from build123d import *

# Parameters (mm, degrees)
F0_R     = 25.4
F0_R_2   = 3.125
F1_DEPTH = 5
F2_R     = 6.031593
F3_DEPTH = 8
F4_R     = 3
F5_DEPTH = 8.001
F8_R     = 1.008959
F9_DEPTH = 8.001


with BuildPart() as f1:
    # F0 (on Top) → F1 (new body)
    with BuildSketch(Plane.XY):
        Circle(F0_R)
        with BuildLine():
            ThreePointArc((-10.88453, -17.158945), (-11.801786, -15.683608), (-11.218679, -14.04716))
            Line((-11.218679, -14.04716), (-6.139343, -9.030124))
            ThreePointArc((-6.139343, -9.030124), (-5.086026, -8.484282), (-3.908805, -8.631157))
            ThreePointArc((-3.908805, -8.631157), (-3.625926, -8.753759), (-3.339207, -8.867092))
            ThreePointArc((-3.339207, -8.867092), (-2.40293, -9.595657), (-2.044091, -10.726433))
            Line((-2.044091, -10.726433), (-2.000038, -17.865646))
            ThreePointArc((-2.000038, -17.865646), (-2.744862, -19.435109), (-4.436681, -19.829732))
            ThreePointArc((-4.436681, -19.829732), (-7.776127, -18.773232), (-10.88453, -17.158945))
        make_face(mode=Mode.SUBTRACT)
        with BuildLine():
            ThreePointArc((-19.829732, -4.436681), (-19.435109, -2.744862), (-17.865646, -2.000038))
            Line((-17.865646, -2.000038), (-10.726433, -2.044091))
            ThreePointArc((-10.726433, -2.044091), (-9.595657, -2.40293), (-8.867092, -3.339207))
            ThreePointArc((-8.867092, -3.339207), (-8.753759, -3.625926), (-8.631157, -3.908805))
            ThreePointArc((-8.631157, -3.908805), (-8.484282, -5.086026), (-9.030124, -6.139343))
            Line((-9.030124, -6.139343), (-14.04716, -11.218679))
            ThreePointArc((-14.04716, -11.218679), (-15.683608, -11.801786), (-17.158945, -10.88453))
            ThreePointArc((-17.158945, -10.88453), (-18.773232, -7.776127), (-19.829732, -4.436681))
        make_face(mode=Mode.SUBTRACT)
        Circle(F0_R_2, mode=Mode.SUBTRACT)
        with BuildLine():
            ThreePointArc((4.436681, -19.829732), (2.744862, -19.435109), (2.000038, -17.865646))
            Line((2.000038, -17.865646), (2.044091, -10.726433))
            ThreePointArc((2.044091, -10.726433), (2.40293, -9.595657), (3.339207, -8.867092))
            ThreePointArc((3.339207, -8.867092), (3.625926, -8.753759), (3.908805, -8.631157))
            ThreePointArc((3.908805, -8.631157), (5.086026, -8.484282), (6.139343, -9.030124))
            Line((6.139343, -9.030124), (11.218679, -14.04716))
            ThreePointArc((11.218679, -14.04716), (11.801786, -15.683608), (10.88453, -17.158945))
            ThreePointArc((10.88453, -17.158945), (7.776127, -18.773232), (4.436681, -19.829732))
        make_face(mode=Mode.SUBTRACT)
        with BuildLine():
            ThreePointArc((17.158945, -10.88453), (15.683608, -11.801786), (14.04716, -11.218679))
            Line((14.04716, -11.218679), (9.030124, -6.139343))
            ThreePointArc((9.030124, -6.139343), (8.484282, -5.086026), (8.631157, -3.908805))
            ThreePointArc((8.631157, -3.908805), (8.753759, -3.625926), (8.867092, -3.339207))
            ThreePointArc((8.867092, -3.339207), (9.595657, -2.40293), (10.726433, -2.044091))
            Line((10.726433, -2.044091), (17.865646, -2.000038))
            ThreePointArc((17.865646, -2.000038), (19.435109, -2.744862), (19.829732, -4.436681))
            ThreePointArc((19.829732, -4.436681), (18.773232, -7.776127), (17.158945, -10.88453))
        make_face(mode=Mode.SUBTRACT)
        with BuildLine():
            ThreePointArc((-17.158945, 10.88453), (-15.683608, 11.801786), (-14.04716, 11.218679))
            Line((-14.04716, 11.218679), (-9.030124, 6.139343))
            ThreePointArc((-9.030124, 6.139343), (-8.484282, 5.086026), (-8.631157, 3.908805))
            ThreePointArc((-8.631157, 3.908805), (-8.753759, 3.625926), (-8.867092, 3.339207))
            ThreePointArc((-8.867092, 3.339207), (-9.595657, 2.40293), (-10.726433, 2.044091))
            Line((-10.726433, 2.044091), (-17.865646, 2.000038))
            ThreePointArc((-17.865646, 2.000038), (-19.435109, 2.744862), (-19.829732, 4.436681))
            ThreePointArc((-19.829732, 4.436681), (-18.773232, 7.776127), (-17.158945, 10.88453))
        make_face(mode=Mode.SUBTRACT)
        with BuildLine():
            ThreePointArc((-10.88453, 17.158945), (-7.776127, 18.773232), (-4.436681, 19.829732))
            ThreePointArc((-4.436681, 19.829732), (-2.744862, 19.435109), (-2.000038, 17.865646))
            Line((-2.000038, 17.865646), (-2.044091, 10.726433))
            ThreePointArc((-2.044091, 10.726433), (-2.40293, 9.595657), (-3.339207, 8.867092))
            ThreePointArc((-3.339207, 8.867092), (-3.625926, 8.753759), (-3.908805, 8.631157))
            ThreePointArc((-3.908805, 8.631157), (-5.086026, 8.484282), (-6.139343, 9.030124))
            Line((-6.139343, 9.030124), (-11.218679, 14.04716))
            ThreePointArc((-11.218679, 14.04716), (-11.801786, 15.683608), (-10.88453, 17.158945))
        make_face(mode=Mode.SUBTRACT)
        with BuildLine():
            ThreePointArc((19.829732, 4.436681), (19.435109, 2.744862), (17.865646, 2.000038))
            Line((17.865646, 2.000038), (10.726433, 2.044091))
            ThreePointArc((10.726433, 2.044091), (9.595657, 2.40293), (8.867092, 3.339207))
            ThreePointArc((8.867092, 3.339207), (8.753759, 3.625926), (8.631157, 3.908805))
            ThreePointArc((8.631157, 3.908805), (8.484282, 5.086026), (9.030124, 6.139343))
            Line((9.030124, 6.139343), (14.04716, 11.218679))
            ThreePointArc((14.04716, 11.218679), (15.683608, 11.801786), (17.158945, 10.88453))
            ThreePointArc((17.158945, 10.88453), (18.773232, 7.776127), (19.829732, 4.436681))
        make_face(mode=Mode.SUBTRACT)
        with BuildLine():
            Line((2.044091, 10.726433), (2.000038, 17.865646))
            ThreePointArc((2.000038, 17.865646), (2.744862, 19.435109), (4.436681, 19.829732))
            ThreePointArc((4.436681, 19.829732), (7.776127, 18.773232), (10.88453, 17.158945))
            ThreePointArc((10.88453, 17.158945), (11.801786, 15.683608), (11.218679, 14.04716))
            Line((11.218679, 14.04716), (6.139343, 9.030124))
            ThreePointArc((6.139343, 9.030124), (5.086026, 8.484282), (3.908805, 8.631157))
            ThreePointArc((3.908805, 8.631157), (3.625926, 8.753759), (3.339207, 8.867092))
            ThreePointArc((3.339207, 8.867092), (2.40293, 9.595657), (2.044091, 10.726433))
        make_face(mode=Mode.SUBTRACT)
    extrude(amount=F1_DEPTH)

    # F2 (on Top) → F3 (join)
    with BuildSketch(Plane.XY):
        Circle(F2_R)
    extrude(amount=F3_DEPTH)

    # F4 (on face) → F5 (cut, through all)
    with BuildSketch(Plane.XY.offset(8)):
        Circle(F4_R)
    extrude(amount=-F5_DEPTH, mode=Mode.SUBTRACT)

    # F6 (on Right) → F7 (revolve, cut)
    with BuildSketch(Plane.YZ):
        Polygon((25.457971, 0.902619), (25.4, 2.402619), (23.4, 2.402619), align=None)
        Polygon((23.4, 2.402619), (25.4, 2.402619), (25.457971, 3.902619), align=None)
    revolve(axis=Axis((0, 0, 8.098846), (0, 0, -1)), mode=Mode.SUBTRACT)

    # F8 (on Top) → F9 (cut, through all)
    with BuildSketch(Plane.XY):
        with Locations((0, 4.377856)):
            Circle(F8_R)
        with Locations((-3.095612, 3.095612)):
            Circle(F8_R)
        with Locations((-4.377856, 0)):
            Circle(F8_R)
        with Locations((-3.095612, -3.095612)):
            Circle(F8_R)
        with Locations((0, -4.377856)):
            Circle(F8_R)
        with Locations((3.095612, -3.095612)):
            Circle(F8_R)
        with Locations((4.377856, 0)):
            Circle(F8_R)
        with Locations((3.095612, 3.095612)):
            Circle(F8_R)
    extrude(amount=F9_DEPTH, mode=Mode.SUBTRACT)


solid = f1.part
Verification items for the finished model (mm, model axes). Give positions to 0.01 mm unless a question says otherwise; leave off trailing zeros. Write each loop counter-clockwise with the first axis right and the second up, starting at its lowest first coordinate (ties: lowest second). Pieces come first, ordered by that corner, then holes. Notation, with made-up numbers: (47.25, 50) - (105.25, 50) arc R27 ccw to (105.25, 89) - close; hole circle Ø8 at (8.5, 79). An arc over 180 degrees is marked (long way). Answer as CSV lines item,"result". Start each with the question number.
1. Thickness scan on line 1 (Y direction, x = 0, z = 5.75); line 2 (Y direction, x = 7, z = 2.25); line 3 (Y direction, x = 14, z = 3.25). Record the ranges inside material, lowest first.
2. Sectioned sample at C-C (z = 6.5). Count the separate pieces of the cut face and the enclosed holes in it, then the cut area to 3 significant figures.
3. Draft check along Y on faces 1 (the face through (-11.57, 8.71, 2.46)), 2 (the face through (5, -5, 5)), 3 (the face through (-5.506, -24.796, 4.422)). Enter one of: pulls with the +Y half, pulls with the -Y half, needs draft (parallel to the pull), parting line crosses it, or undercut.
4. Depth check by flat-ended pin: pin 1 (2.5 mm diameter, centred on x = 3.1, y = 3.1, fed in from -Z); pin 2 (4 mm diameter, centred on x = 4.5, z = 1.5, fed in from +Y); pin 3 (2 mm diameter, centred on x = -6, y = -9, fed in from +Z); pin 4 (1 mm diameter, centred on y = -5.5, z = 4.5, fed in from -X). Enter the tip coordinate at first touch or a pass-through.
5. Sectioned sample at A-A (x = 0). Record the boundary of the cut face in (y, z), then the cut area to 3 significant figures.
Derived:
1,line 1,"-6.03 to -5.39, -3.37 to -3, 3 to 3.37, 5.39 to 6.03"
1,line 2,"-22.55 to -19.08, -9.88 to 9.88, 19.08 to 22.55"
1,line 3,"-20.18 to -11.17, -2.02 to 2.02, 11.17 to 20.18"
2,separate pieces,"1"
2,enclosed holes,"9"
2,area,"60.4 mm²"
3,face 1,"undercut"
3,face 2,"needs draft"
3,face 3,"parting line crosses it"
4,pin 1,"z = 0"
4,pin 2,"y = 25.27"
4,pin 3,"z = 5"
4,pin 4,"x = -24.9"
5,outline,"(-25.4, 0) - (-5.39, 0) - (-5.39, 8) - (-6.03, 8) - (-6.03, 5) - (-25.4, 5) - (-25.4, 3.86) - (-23.4, 2.4) - (-25.4, 0.94) - close; (-3.37, 0) - (-3, 0) - (-3, 8) - (-3.37, 8) - close; (3, 0) - (3.37, 0) - (3.37, 8) - (3, 8) - close; (5.39, 0) - (25.4, 0) - (25.4, 0.94) - (23.4, 2.4) - (25.4, 3.86) - (25.4, 5) - (6.03, 5) - (6.03, 8) - (5.39, 8) - close"
5,area,"204 mm²"
